Autodesk Inventor part; units mm, degrees
ref_plane "YZ Plane" through (0, 0, 0) normal (1, 0, 0) x (0, 1, 0)
ref_plane "XZ Plane" through (0, 0, 0) normal (0, 1, 0) x (-1, 0, 0)
ref_plane "XY Plane" through (0, 0, 0) normal (0, 0, 1) x (1, 0, 0)
sketch "スケッチ1" plane through (0, 0, 0) normal (0, 0, 1) x (1, 0, 0)
  line L0 (-3.5, 3.5) -> (3.5, 3.5)
  line L1 (3.5, 3.5) -> (3.5, -3.5)
  line L2 (3.5, -3.5) -> (-3.5, -3.5)
  line L3 (-3.5, -3.5) -> (-3.5, 3.5)
  line L4 (-3.5, 3.5) -> (3.5, -3.5) construction
  line L5 (3.5, 3.5) -> (-3.5, -3.5) construction
  point P0 (0, 0)
  dimension "d0" = 7
  dimension "d2" = 7
extrude "押し出し1" add sketch "スケッチ1" along normal blind 5
sketch "スケッチ2" plane through (3.5, -3.5, 0) normal (1, 0, 0) x (0, 0, -1)
  line L0 (-5, 0) -> (-5, 7)
  line L1 (0, 0) -> (-5, 0)
  point P0 (0, 3.5)
  point P1 (-2.5, 3.5)
  dimension "d5" = 2.5
  dimension "d6" = 3.5
hole "穴1" at (3.5, 0, 2.5) direction (-1, 0, 0) diameter 2.459 end through all
sketch "スケッチ3" plane through (0, 0, 5) normal (0, 0, 1) x (1, 0, 0)
  line L0 (3.5, 3.5) -> (-3.5, 3.5)
  line L1 (-3.5, 3.5) -> (-3.5, -3.5)
  line L2 (-3.5, -3.5) -> (3.5, -3.5)
  line L3 (3.5, -3.5) -> (3.5, 3.5)
  circle A0 centre (0, 0) radius 3.5
  point P0 (0, 0)
extrude "押し出し2" cut sketch "スケッチ3" against normal blind 5 contours L3 A0 L0 | A0 L1 L0 | L3 L2 A0 | A0 L2 L1
sketch "スケッチ4" plane through (0, 0, 5) normal (0, 0, 1) x (1, 0, 0)
  circle A0 centre (0, 0) radius 3.5
  circle A1 centre (0, 0) radius 1.5
  dimension "d16" = 3
hole "穴2" at (0, 0, 5) at (0, 0, 5) direction (0, 0, -1) diameter 3 end through all
chamfer "面取り1" distance 0.5 angle 45 2 edges at (-3.5, 0, 0) (-3.5, 0, 5)
properties part number "sttopa" material "アルミニウム 2014-T4"
Verification items for the finished model (mm, model axes). Give positions to 0.01 mm unless a question says otherwise; leave off trailing zeros. Write each loop counter-clockwise with the first axis right and the second up, starting at its lowest first coordinate (ties: lowest second). Pieces come first, ordered by that corner, then holes. Notation, with made-up numbers: M 56.5,-38.5 L 83.5,-38.5 A9 cw 83.5,-24.5 Z; hole C 31.5,10.5 d5. An arc over 180 degrees is marked long. One line per question, with ' | ' between items.
1) Thickness scan on line 1 along Z through (x, y) = (-2.8, 0); line 2 along Y through (x, z) = (0, 2.4). Record the ranges inside material, lowest first. Write a range as [from, to].
Result:
line 1: z = [0, 1.27], [3.73, 5] | line 2: y = [-3.5, -1.5], [1.5, 3.5]
2) Section check D-D on z = 4.4. Enter the section's corners in (x, y), plus the area to 3 significant figures.
Result:
outline: C 0,0 d7; hole C 0,0 d3 | area: 31.4 mm2
3) Section check A-A on x = 0. Enter the section's corners in (y, z).
Result:
outline: M -3.5,0.5 L -3,0 L -1.5,0 L -1.5,5 L -3,5 L -3.5,4.5 Z; M 1.5,0 L 3,0 L 3.5,0.5 L 3.5,4.5 L 3,5 L 1.5,5 Z
4) Section check B-B on y = 0. Enter the section's corners in (x, z), plus the area to 3 significant figures.
Result:
outline: M -3.5,0.5 L -3,0 L -1.5,0 L -1.5,1.27 L -3.5,1.27 Z; M -3.5,3.73 L -1.5,3.73 L -1.5,5 L -3,5 L -3.5,4.5 Z; M 1.5,0 L 3,0 L 3.5,0.5 L 3.5,1.27 L 1.5,1.27 Z; M 1.5,3.73 L 3.5,3.73 L 3.5,4.5 L 3,5 L 1.5,5 Z | area: 9.66 mm2
5) Section check C-C on z = 2.15. Enter the section's corners in (x, y), plus the area to 3 significant figures.
Result:
outline: M -3.3,-1.18 A3.5 ccw 3.3,-1.18 L 0.93,-1.18 A1.5 cw -0.93,-1.18 Z; M -3.3,1.18 L -0.93,1.18 A1.5 cw 0.93,1.18 L 3.3,1.18 A3.5 ccw Z | area: 21.5 mm2
6) Mould release check, pull along Y, two halves, no side actions. Record for faces 1 (the flat face through (1.3, -1.3, 5)), 2 (the cylindrical face through (-2.2, -0.05, 3.73)), 3 (the cylindrical face through (1.615, -3.105, 2.528)): released by +Y, released by -Y, zero draft, split by the parting line, or undercut.
Result:
face 1: zero draft | face 2: undercut | face 3: split by the parting line
7) Gauge pin test, flat ends, axial feed: pin 1 Ø1 at (x, z) = (2.5, 2.5) entering from +Y; pin 2 Ø1.8 at (x, y) = (0, 0) entering from +Z; pin 3 Ø1 at (x, z) = (2, 1) entering from +Y. Record the tip position at first contact, or that the pin passes through.
Result:
pin 1: stops at y = 2.87 | pin 2: passes through | pin 3: stops at y = 3.16
